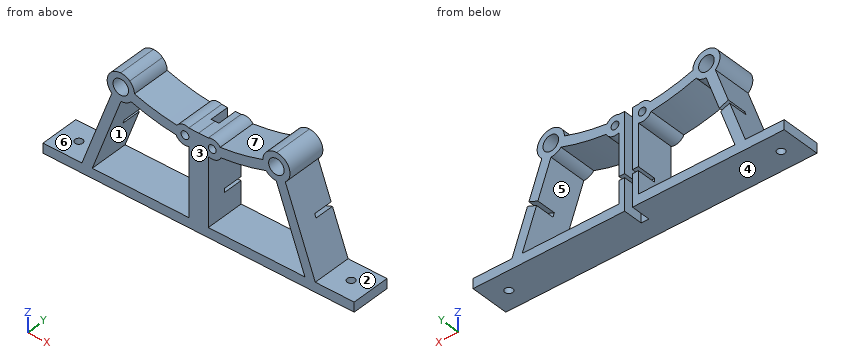
```python
from build123d import *

# Parameters (mm, degrees)
F1_W      = 80
F1_H      = 5
F2_DEPTH  = 10
F3_W      = 5
F3_H      = 151.5
F4_DEPTH  = 10
F5_W      = 21
F5_H      = 23
F6_DEPTH  = 10
F8_DEPTH  = 10
F10_DEPTH = 10
F12_DEPTH = 10
F14_DEPTH = 20
F15_W     = 0.9078182304
F15_H     = 2
F16_DEPTH = 10
F17_R     = 135
F17_R_2   = 133
F18_DEPTH = 10
F19_R     = 7
F19_R_2   = 4
F20_DEPTH = 20
F21_R     = 4
F22_DEPTH = 20.001
F23_R     = 5
F23_R_2   = 2
F24_DEPTH = 20
F26_DEPTH = 20
F28_DEPTH = 20.001
F29_R     = 2
F30_DEPTH = 5.001


# Not quite as in the source:
# - ends of sketch curves that miss each other by under 0.0002 mm in the source are joined


with BuildPart() as f2:
    # F1 (on Front) → F2 (new body)
    with BuildSketch(Plane.XZ):
        with Locations((40, 2.5)):
            Rectangle(F1_W, F1_H)
    extrude(amount=F2_DEPTH)

    # F3 (on Front) → F4 (join, through all)
    with BuildSketch(Plane.XZ):
        with Locations((2.5, 75.75)):
            Rectangle(F3_W, F3_H)
    extrude(amount=F4_DEPTH)

    # F5 (on Front) → F6 (join, through all)
    with BuildSketch(Plane.XZ):
        with Locations((10.5, 151.5)):
            Rectangle(F5_W, F5_H)
    extrude(amount=F6_DEPTH)

    # F7 (on Front) → F8 (join, through all)
    with BuildSketch(Plane.XZ):
        Polygon((60, 5), (9.8688664765, 141.7212732458), (5.1744848971, 140), (55.3056184206, 3.2787267542), align=None)
    extrude(amount=F8_DEPTH)

    # F9 (on face) → F10 (join)
    with BuildSketch(Plane.XZ.offset(10)):
        Polygon((0, 163), (0, 0), (80, 0), (80, 5), (60, 5), (10.5, 140), (21, 140), (21, 163), align=None)
        Polygon((5.1744848971, 140), (54.6744848971, 5), (5, 5), (5, 140), align=None, mode=Mode.SUBTRACT)
    extrude(amount=F10_DEPTH)

    # F11 (on face) → F12 (cut)
    with BuildSketch(Plane(origin=(0, 0, 0), x_dir=(-1, 0, 0), z_dir=(0, 1, 0))):
        Polygon((-2, 0), (0, 0), (0, 140), (-21, 140), (-21, 138), (-2, 138), align=None)
    extrude(amount=-F12_DEPTH, mode=Mode.SUBTRACT)

    # F13 (on face) → F14 (join)
    with BuildSketch(Plane(origin=(0, 0, 0), x_dir=(-1, 0, 0), z_dir=(0, 1, 0))):
        Polygon((-2, 133), (-2, 138), (-11.2333333333, 138), (-13.0666666667, 133), align=None)
    extrude(amount=-F14_DEPTH)

    # F15 (on face) → F16 (join)
    with BuildSketch(Plane.XZ.offset(20)):
        with Locations((5.4539091152, 139)):
            Rectangle(F15_W, F15_H)
    extrude(amount=-F16_DEPTH)

    # F17 (on Front) → F18 (cut)
    with BuildSketch(Plane.XZ):
        with Locations((0, 151.5)):
            Circle(F17_R)
        with Locations((0, 151.5)):
            Circle(F17_R_2, mode=Mode.SUBTRACT)
    extrude(amount=F18_DEPTH, mode=Mode.SUBTRACT)

    # F19 (on Front) → F20 (join, through all)
    with BuildSketch(Plane.XZ):
        with Locations((40.0081513066, 52.2611576598)):
            Circle(F19_R)
        with Locations((40.0081513066, 52.2611576598)):
            Circle(F19_R_2, mode=Mode.SUBTRACT)
    extrude(amount=F20_DEPTH)

    # F21 (on Front) → F22 (cut, through all)
    with BuildSketch(Plane.XZ):
        with Locations((40.0081513066, 52.2611576598)):
            Circle(F21_R)
    extrude(amount=F22_DEPTH, mode=Mode.SUBTRACT)

    # F23 (on Front) → F24 (join, through all)
    with BuildSketch(Plane.XZ):
        with Locations((7, 44.7292174797)):
            Circle(F23_R)
        with Locations((7, 44.7292174797)):
            Circle(F23_R_2, mode=Mode.SUBTRACT)
    extrude(amount=F24_DEPTH)

    # F25 (on Front) → F26 (join, through all)
    with BuildSketch(Plane.XZ):
        with BuildLine():
            Line((8.7843409429, 47.3698633718), (8.9944926401, 44.8787117779))
            ThreePointArc((8.9944926401, 44.8787117779), (22.8274604253, 46.9633698145), (36.2703225327, 50.8348933176))
            Line((36.2703225327, 50.8348933176), (35.4228850903, 53.1868817915))
            ThreePointArc((35.4228850903, 53.1868817915), (22.294150224, 49.4058235462), (8.7843409429, 47.3698633718))
        make_face()
        with BuildLine():
            ThreePointArc((36.2703225327, 50.8348933176), (22.8274604253, 46.9633698145), (8.9944055882, 44.8787044343))
            Line((8.9944055882, 44.8787044343), (9.2046443373, 42.3875601839))
            ThreePointArc((9.2046443373, 42.3875601839), (23.3608559764, 44.5209347206), (37.117759975, 48.4829048437))
            Line((37.117759975, 48.4829048437), (36.2703225327, 50.8348933176))
        make_face()
    extrude(amount=F26_DEPTH)

    # F27 (on Front) → F28 (cut, through all)
    with BuildSketch(Plane.XZ):
        with BuildLine():
            ThreePointArc((5, 49.3117931746), (8.3573933592, 49.5414397593), (11.0998968806, 47.5911828128))
            ThreePointArc((11.0998968806, 47.5911828128), (22.1823046987, 49.3814641789), (33.0087181874, 52.3502419386))
            ThreePointArc((33.0087181874, 52.3502419386), (38.6064619078, 59.1193838757), (46.4113234148, 55.0894764101))
            ThreePointArc((46.4113234148, 55.0894764101), (104.3190443402, 175.3020374745), (0, 258.5))
            Line((0, 258.5), (0, 253.8104570129))
            ThreePointArc((0, 253.8104570129), (-102.2798898997, 148.9992528562), (5, 49.3117931746))
        make_face()
    extrude(amount=F28_DEPTH, mode=Mode.SUBTRACT)

    # F29 (on face) → F30 (cut, through all)
    with BuildSketch(Plane.XY.offset(5)):
        with Locations((70, -10)):
            Circle(F29_R)
    extrude(amount=-F30_DEPTH, mode=Mode.SUBTRACT)

    # F31: F2 across plane


with BuildPart() as f2_1:
    add(f2.part)
    add(f2.part.mirror(Plane.YZ))


solid = f2_1.part
```
The listing builds one solid part. Answer for the finished solid, in the listing's coordinates (mm). Face numbers are marked on the shaded views. A direction names the side the tool comes from. Give positions to 0.01 mm unless a question says otherwise; leave off trailing zeros. Order: outer loops, then holes, each group sorted by start corner. A loop starts at its lowest first (then second) coordinate and runs counter-clockwise, first axis right, second up. Notation, with made-up numbers: (-16.5, 70) -> (13.5, 70) arc R31 cw to (13.5, 101) -> close; hole circle Ø3 at (-5, -4.5). An arc over 180 degrees is marked (long way). Answer as CSV lines item,"result". Start each with the question number.
Q1. A cutting plane is placed at B-B (z = 31.5). Determine the outline of the cut face in (x, y).
Q2. Determine the mould class of the marked faces 1, 2, 3 and 4 for opening direction Z: pulls with the +Z half, pulls with the -Z half, needs draft (parallel to the pull), parting line crosses it, or undercut.
Q3. A cutting plane is placed at C-C (x = 7). Determine the outline of the cut face in (y, z).
Q4. A cutting plane is placed at D-D (y = -5.75). Count the separate pieces of the cut face and the enclosed holes in it, then the cut area to 3 significant figures.
Q5. A cutting plane is placed at A-A (x = 70). Determine the outline of the cut face in (y, z).
Q6. Find the intervals of material crossed by L1, parallel to Z at x = 7, y = -10; L2, parallel to X at y = -7.75, z = 12; L3, parallel to Z at x = 38, y = -4.25, in increasing order.
Q7. Which of the six approach directions +Z, -Z, +X, -X, +Y, -Y give full straight-line access (tool end or side, diameter ignored) to the marked faces 5, 6 and 7?
Q8. Given pin 1 (5 mm diameter, centred on y = -6, z = 37.5, fed in from -X); pin 2 (6 mm diameter, centred on y = -13, z = 14.5, fed in from +X); pin 3 (6 mm diameter, centred on x = 73.5, y = -9.5, fed in from +Z), each flat-ended and moving along its own axis, determine where each tip first touches the part or whether it passes through.
Results found:
1,outline,"(-50.28, -20) -> (-44.96, -20) -> (-44.96, 0) -> (-50.28, 0) -> close; (-5, -20) -> (5, -20) -> (5, 0) -> (2, 0) -> (2, -10) -> (-2, -10) -> (-2, 0) -> (-5, 0) -> close; (44.96, -20) -> (50.28, -20) -> (50.28, 0) -> (44.96, 0) -> close"
2,face 1,"undercut"
2,face 2,"pulls with the +Z half"
2,face 3,"needs draft"
2,face 4,"pulls with the -Z half"
3,outline,"(-20, 0) -> (0, 0) -> (0, 5) -> (-20, 5) -> close; (-20, 39.73) -> (0, 39.73) -> (0, 42.73) -> (-20, 42.73) -> close; (-20, 46.73) -> (0, 46.73) -> (0, 49.73) -> (-20, 49.73) -> close"
4,separate pieces,"4"
4,enclosed holes,"4"
4,area,"1,970 mm2"
5,outline,"(-20, 0) -> (-12, 0) -> (-12, 5) -> (-20, 5) -> close; (-8, 0) -> (0, 0) -> (0, 5) -> (-8, 5) -> close"
6,L1,"0 to 5, 39.73 to 42.73, 46.73 to 49.73"
6,L2,"-57.43 to -52.11, -5 to -2, 2 to 5, 52.11 to 57.43"
6,L3,"0 to 5, 45.56 to 48.8, 55.72 to 58.97"
7,face 5,"+Y, -Y"
7,face 6,"+Z, -X, +Y, -Y"
7,face 7,"+Z, +Y, -Y"
8,pin 1,"x = -49"
8,pin 2,"x = 57.62"
8,pin 3,"z = 5"
